from build123d import *

# Parameters (mm, degrees)
SKETCH_1_R      = 1.5
SKETCH_1_R_2    = 3.5
EXTRUDE_1_DEPTH = 4
FILLET_1_R      = 3


with BuildPart() as part:
    # 草图1 → 凸台-拉伸1 (new body)
    with BuildSketch(Plane.XY):
        Polygon((-10, 10), (-25, 10), (-25, -10), (-10, -10), (-10, -25), (10, -25), (10, -10), (25, -10), (25, 10), (10, 10), (10, 25), (-10, 25), align=None)
        with Locations((-20, -5)):
            Circle(SKETCH_1_R, mode=Mode.SUBTRACT)
        with Locations((-20, 5)):
            Circle(SKETCH_1_R, mode=Mode.SUBTRACT)
        with Locations((5, 5)):
            Circle(SKETCH_1_R, mode=Mode.SUBTRACT)
        with Locations((-5, -5)):
            Circle(SKETCH_1_R, mode=Mode.SUBTRACT)
        with Locations((5, -5)):
            Circle(SKETCH_1_R, mode=Mode.SUBTRACT)
        Circle(SKETCH_1_R_2, mode=Mode.SUBTRACT)
        with Locations((-5, 5)):
            Circle(SKETCH_1_R, mode=Mode.SUBTRACT)
        with Locations((5, 20)):
            Circle(SKETCH_1_R, mode=Mode.SUBTRACT)
        with Locations((-5, 20)):
            Circle(SKETCH_1_R, mode=Mode.SUBTRACT)
        with Locations((20, 5)):
            Circle(SKETCH_1_R, mode=Mode.SUBTRACT)
        with Locations((20, -5)):
            Circle(SKETCH_1_R, mode=Mode.SUBTRACT)
        with Locations((5, -20)):
            Circle(SKETCH_1_R, mode=Mode.SUBTRACT)
        with Locations((-5, -20)):
            Circle(SKETCH_1_R, mode=Mode.SUBTRACT)
    extrude(amount=EXTRUDE_1_DEPTH)

    # 圆角1
    fillet_1_edges = [part.edges().sort_by_distance(p)[0] for p in [
        (25, 10, 2),
        (25, -10, 2),
        (10, -10, 2),
        (10, -25, 2),
        (-10, -25, 2),
        (-10, -10, 2),
        (-25, -10, 2),
        (-25, 10, 2),
        (-10, 10, 2),
        (-10, 25, 2),
        (10, 25, 2),
        (10, 10, 2),
    ]]
    fillet(fillet_1_edges, radius=FILLET_1_R)


solid = part.part
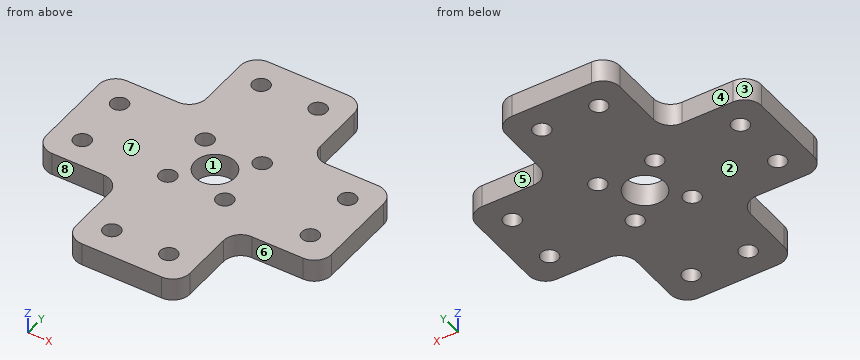
For this review, take the finished solid that the model builds, in its own axes (mm). Face numbers are marked on the shaded views. A direction names the side the tool comes from. Coordinates: 2 decimals unless noted, no trailing zeros. Loops run counter-clockwise (first coordinate to the right, second up) from the corner with the lowest first, then second, coordinate; pieces in that order, holes last. Notation, with made-up numbers: (38.25, 51) - (47.25, 51) arc R16 ccw to (47.25, 55) - close; hole circle Ø11 at (71, 35). An arc over 180 degrees is marked (long way). Return JSON: item names as keys, results as strings.
Item 1: Take a section at D-D (x = 0). Give the boundary of the cut face in (y, z).
Determined:
{"outline": "(-25, 0) - (-3.5, 0) - (-3.5, 4) - (-25, 4) - close; (3.5, 0) - (25, 0) - (25, 4) - (3.5, 4) - close"}
Item 2: Mouldability with a two-part tool opening along X and no side actions: class the marked faces 1, 2 and 3 as pulls with the +X half, pulls with the -X half, needs draft (parallel to the pull), parting line crosses it, or undercut.
Determined:
{"face 1": "undercut", "face 2": "needs draft", "face 3": "pulls with the -X half"}
Item 3: For line 1 (Y direction, x = 20, z = 3.2); line 2 (Y direction, x = -5, z = 1.9); line 3 (Y direction, x = 19.5, z = 0.55), list the stretches that pass through material, from the lowest coordinate up.
Determined:
{"line 1": "y = -10 to -6.5, -3.5 to 3.5, 6.5 to 10", "line 2": "y = -25 to -21.5, -18.5 to -6.5, -3.5 to 3.5, 6.5 to 18.5, 21.5 to 25", "line 3": "y = -10 to -6.41, -3.59 to 3.59, 6.41 to 10"}
Item 4: Take a section at A-A (y = 5). Give the boundary of the cut face in (x, z).
Determined:
{"outline": "(-25, 0) - (-21.5, 0) - (-21.5, 4) - (-25, 4) - close; (-18.5, 0) - (-6.5, 0) - (-6.5, 4) - (-18.5, 4) - close; (-3.5, 0) - (3.5, 0) - (3.5, 4) - (-3.5, 4) - close; (6.5, 0) - (18.5, 0) - (18.5, 4) - (6.5, 4) - close; (21.5, 0) - (25, 0) - (25, 4) - (21.5, 4) - close"}
Item 5: Insertion check: pin 1 (1.8 mm diameter, centred on x = -5, y = 5, fed in from -Z); pin 2 (1.2 mm diameter, centred on y = -16.5, z = 3, fed in from +X). Each pin has a flat end and moves straight along its axis. Give the tip position at first contact, or say it passes through.
Determined:
{"pin 1": "passes through", "pin 2": "stops at x = 10"}
Item 6: For the marked faces 4, 5, 6, 7 and 8, list the 3-axis set-ups (+Z, -Z, +X, -X, +Y, -Y) from which the entire face can be reached by the end or side of a thin tool; tool diameter is ignored.
Determined:
{"face 4": "+Z, -Z, -X, +Y", "face 5": "+Z, -Z, +X, +Y", "face 6": "+Z, -Z, +X, -Y", "face 7": "+Z, +X, -X, +Y, -Y", "face 8": "+Z, -Z, -X, -Y"}
Item 7: Take a section at B-B (x = 20). Give the boundary of the cut face in (y, z).
Determined:
{"outline": "(-10, 0) - (-6.5, 0) - (-6.5, 4) - (-10, 4) - close; (-3.5, 0) - (3.5, 0) - (3.5, 4) - (-3.5, 4) - close; (6.5, 0) - (10, 0) - (10, 4) - (6.5, 4) - close"}
